CAD build for the part. Positions are in the model's coordinates, mm. Face numbers are marked on the shaded views. Round coordinates to 2 decimals unless told otherwise and drop trailing zeros. Order: outer loops, then holes, each group sorted by start corner. A loop starts at its lowest first (then second) coordinate and runs counter-clockwise, first axis right, second up. Notation, with made-up numbers: (77.25, -11.5) -> (95.25, -11.5) arc R18 cw to (95.25, 7.5) -> close; hole circle Ø7 at (5, 47). An arc over 180 degrees is marked (long way). Return JSON: item names as keys, results as strings. Group by question number.
Q1. Cut at C-C (y = -19.5). Write the cut outline in (x, z), then the cut area to 3 significant figures.
Q2. Cut at D-D (z = -38). Write the cut outline in (x, y).
Q3. Probe line 1 along Z through (x, y) = (-0.5, -14); line 2 along X through (y, z) = (-9, -5); line 3 along X through (y, z) = (12, 16). List the from-to ranges inside material, lowest first.
Q4. Mould opens along Z. For the marked faces 1, 2, 3 and 4 say: +Z half, -Z half, draft (parallel to the pull), parting line (faces both ways), or undercut.
Q5. Cut at A-A (z = 0). Write the cut outline in (x, y), then the cut area to 3 significant figures.
Q6. Flat gauge pin, fed straight in: pin 1 (12 mm diameter, centred on x = 20.5, y = 15.5, fed in from -Z). Where does the tip first touch, or does it go through?
Q7. Cut at B-B (x = 0). Write the cut outline in (y, z), then the cut area to 3 significant figures.
from build123d import *

# Parameters (mm, degrees)
F0_W     = 127
F0_H     = 50.8
F1_DEPTH = 63.5
F2_R     = 50.8
F3_R     = 31.75
F4_DEPTH = 50.801


with BuildPart() as f1:
    # F0 (on Top) → F1 (new body, symmetric)
    with BuildSketch(Plane.XY):
        Rectangle(F0_W, F0_H)
    extrude(amount=F1_DEPTH, both=True)

    # F2
    f2_edges = [f1.edges().sort_by_distance(p)[0] for p in [
        (63.5, 0, -63.5),
    ]]
    fillet(f2_edges, radius=F2_R)

    # F3 (on face) → F4 (cut, through all)
    with BuildSketch(Plane.XZ.offset(25.4)):
        Circle(F3_R)
    extrude(amount=-F4_DEPTH, mode=Mode.SUBTRACT)


solid = f1.part
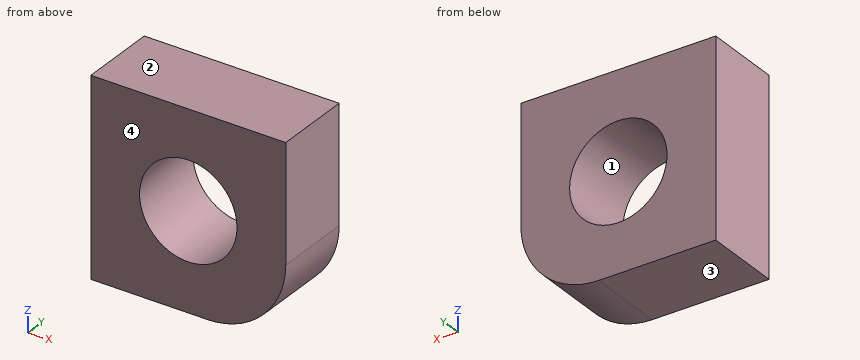
Solution:
{
 "1": {"outline": "(-63.5, -63.5) -> (12.7, -63.5) arc R50.8 ccw to (63.5, -12.7) -> (63.5, 63.5) -> (-63.5, 63.5) -> close; hole circle Ø63.5 at (0, 0)", "area": "12,400 mm²"},
 "2": {"outline": "(-63.5, -25.4) -> (56.75, -25.4) -> (56.75, 25.4) -> (-63.5, 25.4) -> close"},
 "3": {"line 1": "z = -63.5 to -31.75, 31.75 to 63.5", "line 2": "x = -63.5 to -31.35, 31.35 to 63.5", "line 3": "x = -63.5 to -27.42, 27.42 to 63.5"},
 "4": {"face 1": "undercut", "face 2": "+Z half", "face 3": "-Z half", "face 4": "draft"},
 "5": {"outline": "(-63.5, -25.4) -> (-31.75, -25.4) -> (-31.75, 25.4) -> (-63.5, 25.4) -> close; (31.75, -25.4) -> (63.5, -25.4) -> (63.5, 25.4) -> (31.75, 25.4) -> close", "area": "3,230 mm²"},
 "6": {"pin 1": "stops at z = -63.47"},
 "7": {"outline": "(-25.4, -63.5) -> (25.4, -63.5) -> (25.4, -31.75) -> (-25.4, -31.75) -> close; (-25.4, 31.75) -> (25.4, 31.75) -> (25.4, 63.5) -> (-25.4, 63.5) -> close", "area": "3,230 mm²"}
}
